Geometry check sheet. Reference: the model listing, model coordinates, mm. Face numbers are marked on the shaded views. Give positions to 0.01 mm unless a question says otherwise; leave off trailing zeros. Write each loop counter-clockwise with the first axis right and the second up, starting at its lowest first coordinate (ties: lowest second). Pieces come first, ordered by that corner, then holes. Notation, with made-up numbers: (10, -16) - (26, -16) arc R14 cw to (26, -9) - close; hole circle Ø3 at (88.25, 26). An arc over 180 degrees is marked (long way). One line per question, with ' | ' between items. Start each with the question number.
Q1. Gauge pin test, flat ends, axial feed: P1, Ø3.5, axis at x = -44.5, z = -35.5, coming from the +Y side; P2, Ø1.5, axis at y = 1, z = 21, coming from the +X side; P3, Ø10, axis at x = -45.5, z = 38, coming from the +Y side; P4, Ø1.5, axis at x = 29, z = -28, coming from the -Y side. Record the tip position at first contact, or that the pin passes through.
Q2. Section check B-B on y = 5.5. Record the boundary of the cut face in (x, z).
Q3. Section check A-A on z = 36.75. Record the boundary of the cut face in (x, y).
Q4. Section check D-D on z = 21.5. Record the boundary of the cut face in (x, y), and give its area (3 significant figures).
Q5. Section check C-C on x = 17.5. Record the boundary of the cut face in (y, z), and give its area (3 significant figures).
Q6. Thickness scan on L1, parallel to X at y = 2.3, z = -36.85; L2, parallel to X at y = 1.15, z = 36.75; L3, parallel to Z at x = -44.1, y = 2.65. Record the ranges inside material, lowest first. Write a range as [from, to].
Q7. Release check for a two-part mould opening along X. For the marked faces 1 and 2 record: +X half, -X half, draft (parallel to the pull), parting line (faces both ways), or undercut.
Autodesk Inventor part; units mm, degrees
ref_plane "YZ Plane" through (0, 0, 0) normal (1, 0, 0) x (0, 1, 0)
ref_plane "XZ Plane" through (0, 0, 0) normal (0, 1, 0) x (-1, 0, 0)
ref_plane "XY Plane" through (0, 0, 0) normal (0, 0, 1) x (1, 0, 0)
sketch "Boceto1" plane through (0, 0, 0) normal (0, 1, 0) x (-1, 0, 0)
  line L0 (-31.6, 39.35) -> (-31.6, -39.25)
  line L1 (-31.6, -39.25) -> (31.5, -39.25)
  line L2 (31.5, -39.25) -> (31.5, 39.35)
  line L3 (31.5, 39.35) -> (-31.6, 39.35)
  line L4 (-31.6, 39.35) -> (31.5, -39.25) construction
  line L5 (-31.6, -39.25) -> (31.5, 39.35) construction
  line L6 (36.5, 44.35) -> (36.5, -44.25)
  line L7 (36.5, -44.25) -> (-36.6, -44.25)
  line L8 (-36.6, -44.25) -> (-36.6, 44.35)
  line L9 (-36.6, 44.35) -> (36.5, 44.35)
  point P0 (0, 0)
  point P1 (-0.05, 0.05)
  dimension "d0" = 78.6
  dimension "d1" = 63.1
  dimension "d2" = 5
extrude "Extrusión1" add sketch "Boceto1" along normal blind 2 contours L3 L2 L1 L0
sketch "Boceto2" plane through (0, 0, 0) normal (0, 1, 0) x (-1, 0, 0)
  line L0 (-31.6, 39.35) -> (-31.6, -39.25)
  line L1 (-31.6, -39.25) -> (31.5, -39.25)
  line L2 (31.5, -39.25) -> (31.5, 39.35)
  line L3 (31.5, 39.35) -> (-31.6, 39.35)
  line L4 (-31.6, 39.35) -> (31.5, -39.25) construction
  line L5 (-31.6, -39.25) -> (31.5, 39.35) construction
  line L6 (36.5, 44.35) -> (36.5, -44.25)
  line L7 (36.5, -44.25) -> (-36.6, -44.25)
  line L8 (-36.6, -44.25) -> (-36.6, 44.35)
  line L9 (-36.6, 44.35) -> (36.5, 44.35)
  point P0 (0, 0)
  point P1 (0, 0)
  point P2 (-0.05, 0.05)
  dimension "d5" = 78.6
  dimension "d6" = 63.1
  dimension "d7" = 5
extrude "Extrusión2" add sketch "Boceto2" along normal blind 7
sketch "Boceto3" plane through (0, 0, 0) normal (0, 1, 0) x (-1, 0, 0)
  circle A0 centre (44, 36.85) radius 6.1
  line L0 (36.5, 44.35) -> (-36.6, 44.35)
  line L1 (36.5, 44.35) -> (51.5, 44.35)
  line L2 (51.5, 44.35) -> (51.5, 29.35)
  line L3 (51.5, 29.35) -> (36.5, 29.35)
  line L4 (36.5, 29.35) -> (36.5, 44.35)
  line L5 (36.5, -44.25) -> (36.5, 44.35)
  line L6 (36.5, 0.05) -> (47.8738, 0.05)
  line L7 (-0.05, 44.35) -> (-0.05, 26.6285)
  circle A1 centre (44, -36.75) radius 6.1
  line L8 (36.5, -44.25) -> (51.5, -44.25)
  line L9 (51.5, -44.25) -> (51.5, -29.25)
  line L10 (51.5, -29.25) -> (36.5, -29.25)
  line L11 (36.5, -29.25) -> (36.5, -44.25)
  circle A2 centre (-44.1, 36.85) radius 6.1
  line L12 (-36.6, 44.35) -> (-51.6, 44.35)
  line L13 (-51.6, 44.35) -> (-51.6, 29.35)
  line L14 (-51.6, 29.35) -> (-36.6, 29.35)
  line L15 (-36.6, 29.35) -> (-36.6, 44.35)
  circle A3 centre (-44.1, -36.75) radius 6.1
  line L16 (-36.6, -44.25) -> (-51.6, -44.25)
  line L17 (-51.6, -44.25) -> (-51.6, -29.25)
  line L18 (-51.6, -29.25) -> (-36.6, -29.25)
  line L19 (-36.6, -29.25) -> (-36.6, -44.25)
  line L20 (44, 29.35) -> (36.5, 29.35)
  line L21 (36.5, 29.35) -> (36.5, -29.25)
  line L22 (36.5, -29.25) -> (44, -29.25)
  line L23 (44, -29.25) -> (44, 29.35)
  line L24 (-36.6, 0.05) -> (-47.9738, 0.05)
  line L25 (-36.6, 29.35) -> (-36.6, -29.25)
  line L26 (-44.1, -29.25) -> (-44.1, 29.35)
  point P0 (0, 0)
  dimension "d10" = 12.2
  dimension "d11" = 15
  dimension "d12" = 15
extrude "Extrusión3" add sketch "Boceto3" along normal blind 3 contours A0 | L15 L14 L13 L12 | L1 L2 L3 L4 | L3 L23 L6 L5 | L6 L23 L10 L5 | L25 L24 L26 L14 | L10 L9 L8 L5 | L25 L18 L26 L24 | L19 L16 L17 L18 | A1 | A2 | A3
sketch "Boceto4" plane through (0, 3, 0) normal (0, 1, 0) x (1, 0, 0)
  circle A0 centre (44, 36.85) radius 6.1
  line L0 (36.5, 44.35) -> (-36.6, 44.35)
  line L1 (36.5, 44.35) -> (51.5, 44.35)
  line L2 (51.5, 44.35) -> (51.5, 29.35)
  line L3 (51.5, 29.35) -> (36.5, 29.35)
  line L4 (36.5, 29.35) -> (36.5, 44.35)
  line L5 (36.5, -44.25) -> (36.5, 44.35)
  line L6 (36.5, 0.05) -> (47.8738, 0.05)
  line L7 (-0.05, 44.35) -> (-0.05, 26.6285)
  circle A1 centre (44, -36.75) radius 6.1
  line L8 (36.5, -44.25) -> (51.5, -44.25)
  line L9 (51.5, -44.25) -> (51.5, -29.25)
  line L10 (51.5, -29.25) -> (36.5, -29.25)
  line L11 (36.5, -29.25) -> (36.5, -44.25)
  line L12 (-51.6, 29.35) -> (-36.6, 29.35)
  circle A2 centre (-44.1, 36.85) radius 6.1
  line L13 (-36.6, 44.35) -> (-51.6, 44.35)
  line L14 (-36.6, 29.35) -> (-36.6, 44.35)
  line L15 (-51.6, 44.35) -> (-51.6, 29.35)
  line L16 (-51.6, -29.25) -> (-36.6, -29.25)
  circle A3 centre (-44.1, -36.75) radius 6.1
  line L17 (-36.6, -29.25) -> (-36.6, -44.25)
  line L18 (-51.6, -44.25) -> (-51.6, -29.25)
  line L19 (-36.6, -44.25) -> (-51.6, -44.25)
  point P0 (0, 0)
  point P1 (0, 0)
  dimension "d15" = 12.2
  dimension "d16" = 15
  dimension "d17" = 15
extrude "Extrusión4" cut sketch "Boceto4" against normal blind 1 contours A0 | A1 | A2 | A3
sketch "Boceto5" plane through (-44.1, 2, 36.75) normal (0, 1, 0) x (1, 0, 0)
  circle A0 centre (0, 0) radius 2.25
  line L0 (7.6, 66) -> (7.6, 7.4)
  line L1 (7.6, 36.7) -> (1.3256, 36.7)
  line L2 (44.1, -8.1109) -> (44.1, -20.0015)
  circle A1 centre (0, 73.4) radius 2.25
  circle A2 centre (88.2, 0) radius 2.25
  circle A3 centre (88.2, 73.4) radius 2.25
  point P0 (44.1, 36.75)
  dimension "d20" = 4.5
extrude "Extrusión5" cut sketch "Boceto5" against normal blind 2
properties part number "battery_pack_base"
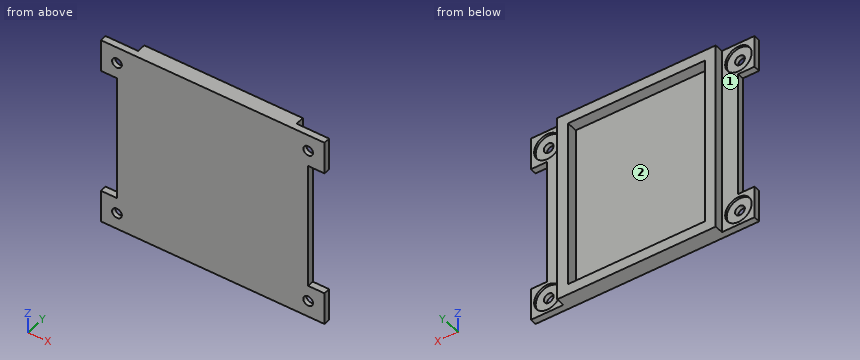
Working result:
1) P1: stops at y = 2 | P2: stops at x = 44.1 | P3: stops at y = 3 | P4: stops at y = 0
2) outline: (-36.5, -44.25) - (36.6, -44.25) - (36.6, 44.35) - (-36.5, 44.35) - close; hole (-31.5, -39.25) - (31.6, -39.25) - (31.6, 39.35) - (-31.5, 39.35) - close
3) outline: (-51.5, 0) - (-46.35, 0) - (-46.35, 2) - (-50.2, 2) - (-50.2, 3) - (-51.5, 3) - close; (-41.85, 0) - (41.85, 0) - (41.85, 2) - (37.9, 2) - (37.9, 3) - (36.6, 3) - (36.6, 7) - (31.6, 7) - (31.6, 2) - (-31.5, 2) - (-31.5, 7) - (-36.5, 7) - (-36.5, 3) - (-38, 3) - (-38, 2) - (-41.85, 2) - close; (46.35, 0) - (51.6, 0) - (51.6, 3) - (50.1, 3) - (50.1, 2) - (46.35, 2) - close
4) outline: (-44, 0) - (44.1, 0) - (44.1, 3) - (36.6, 3) - (36.6, 7) - (31.6, 7) - (31.6, 2) - (-31.5, 2) - (-31.5, 7) - (-36.5, 7) - (-36.5, 3) - (-44, 3) - close | area: 241 mm2
5) outline: (0, -44.25) - (7, -44.25) - (7, -39.25) - (2, -39.25) - (2, 39.35) - (7, 39.35) - (7, 44.35) - (0, 44.35) - close | area: 227 mm2
6) L1: x = [-51.5, -50.2], [-38, -31.5], [31.6, 37.9], [50.1, 51.6] | L2: x = [-51.5, -46.35], [-41.85, 41.85], [46.35, 51.6] | L3: z = [-44.25, -42.95], [-30.75, -29.25], [29.35, 30.65], [42.85, 44.35]
7) face 1: draft | face 2: undercut
